Build history of the part. All positions in model axes, mm. A direction names the side the tool comes from. Round coordinates to 2 decimals unless told otherwise and drop trailing zeros. Loops run counter-clockwise (first coordinate to the right, second up) from the corner with the lowest first, then second, coordinate; pieces in that order, holes last. Notation, with made-up numbers: (45, 37.25) - (59, 37.25) arc R26 cw to (59, 59.25) - close; hole circle Ø3 at (88.5, -11.5). An arc over 180 degrees is marked (long way). Use a Markdown table: item, result.
from build123d import *

# Parameters (mm, degrees)
BOSS_EXTRUDE1_DEPTH = 10
SKETCH3_R           = 2.9999999999999973
CUT_EXTRUDE1_DEPTH  = 10
FILLET3_R           = 2
SKETCH4_R           = 1.4999999999999998
CUT_EXTRUDE2_DEPTH  = 10
SKETCH5_R           = 1.5000000000000002
CUT_EXTRUDE3_DEPTH  = 10


with BuildPart() as part:
    # Sketch2 → Boss-Extrude1 (new body)
    with BuildSketch(Plane(origin=(0, 0, 0), x_dir=(1, 0, 0), z_dir=(0, 1, 0))):
        Polygon((32.000000000000014, -27.000000000000004), (39.000000000000014, -27.000000000000004), (39.00000000000001, 18.000000000000004), (-18, 18), (-18, -13), (-12.999999999999998, -13), (-12.999999999999998, 13), (13.000000000000002, 13), (32, 13), align=None)
    extrude(amount=BOSS_EXTRUDE1_DEPTH)

    # Sketch3 → Cut-Extrude1 (cut)
    with BuildSketch(Plane(origin=(39.00000000000001, 0, -6.01e-15), x_dir=(0, 0, -1), z_dir=(1, 0, 0))):
        with Locations((-21, 5)):
            Circle(SKETCH3_R)
    extrude(amount=-CUT_EXTRUDE1_DEPTH, mode=Mode.SUBTRACT)

    # Fillet3
    fillet3_edges = [part.edges().sort_by_distance(p)[0] for p in [
        (-15.5, 0, 13),
        (-18, 0, -2.5),
        (10.500000000000004, 0, -18),
        (39.000000000000014, 0, 4.5),
        (35.500000000000014, 0, 27.000000000000004),
        (10.500000000000004, 10, -18),
        (-18, 5, 13),
        (-18, 5, -18),
        (39.00000000000001, 5, -18.000000000000004),
        (39.000000000000014, 5, 27.000000000000004),
        (-18, 10, -2.5),
        (-15.5, 10, 13),
        (35.500000000000014, 10, 27.000000000000004),
        (39.000000000000014, 10, 4.5),
    ]]
    fillet(fillet3_edges, radius=FILLET3_R)

    # Sketch4 → Cut-Extrude2 (cut)
    with BuildSketch(Plane(origin=(-1.1e-15, 0, -18), x_dir=(-1, 0, 6e-17), z_dir=(-6e-17, 0, -1))):
        with Locations((0.5000000000000004, 5)):
            Circle(SKETCH4_R)
    extrude(amount=-CUT_EXTRUDE2_DEPTH, mode=Mode.SUBTRACT)

    # Sketch5 → Cut-Extrude3 (cut)
    with BuildSketch(Plane.ZY.offset(18)):
        with Locations((3.47e-15, 5)):
            Circle(SKETCH5_R)
    extrude(amount=-CUT_EXTRUDE3_DEPTH, mode=Mode.SUBTRACT)


solid = part.part
Q1. Cut at C-C, the plane y = 5. List the corners of the cut face in (x, z), plus the area to 3 significant figures.
Results found:
| item | result |
|---|---|
| outline | (-18, -16) arc R2 ccw to (-16, -18) - (-2, -18) - (-2, -13) - (-13, -13) - (-13, -1.5) - (-18, -1.5) - close; (-18, 1.5) - (-13, 1.5) - (-13, 13) - (-16, 13) arc R2 ccw to (-18, 11) - close; (1, -18) - (37, -18) arc R2 ccw to (39, -16) - (39, 18) - (32, 18) - (32, -13) - (1, -13) - close; (32, 24) - (39, 24) - (39, 25) arc R2 ccw to (37, 27) - (32, 27) - close |
| area | 620 mm2 |
Q2. Cut at A-A, the plane z = -3.5. List the corners of the cut face in (x, y).
Results found:
| item | result |
|---|---|
| outline | (-18, 2) arc R2 ccw to (-16, 0) - (-13, 0) - (-13, 10) - (-16, 10) arc R2 ccw to (-18, 8) - close; (32, 0) - (37, 0) arc R2 ccw to (39, 2) - (39, 8) arc R2 ccw to (37, 10) - (32, 10) - close |
Q3. Probe line 1 (X direction, y = 6, z = 6); line 2 (Z direction, x = 16.5, y = 4.75); line 3 (X direction, y = 2.5, z = 19). List the from-to ranges inside material, lowest first.
Results found:
| item | result |
|---|---|
| line 1 | x = -18 to -13, 32 to 39 |
| line 2 | z = -18 to -13 |
| line 3 | x = 32 to 39 |
Q4. Drop flat-ended pins along their axis: pin 1 (6 mm diameter, centred on x = -7, z = -8.5, fed in from +Y); pin 2 (2.5 mm diameter, centred on x = -14.5, y = 5.5, fed in from +Z); pin 3 (2 mm diameter, centred on y = 3.5, z = 13, fed in from -X); pin 4 (5 mm diameter, centred on x = 15, y = 3.5, fed in from +Z). Give the stop position or say it passes through.
Results found:
| item | result |
|---|---|
| pin 1 | passes through |
| pin 2 | stops at z = 13 |
| pin 3 | stops at x = -17.73 |
| pin 4 | stops at z = -13 |
Q5. Which spindle directions (+Z, -Z, +X, -X, +Y, -Y) get a long thin tool onto all of the face, cutting with end or side? Do faces 1 (the face through (-15.5, 4.1, -1.2)), 2 (the face through (36, 5, 24)), 3 (the face through (38.43, 0.6, 4.21)), 4 (the face through (9, 5, -13)), 5 (the face through (-15, 5, 13)). Say none if no direction does.
Results found:
| item | result |
|---|---|
| face 1 | -X |
| face 2 | +X, -X |
| face 3 | +Z, -Z, +X, -Y |
| face 4 | +Z, +Y, -Y |
| face 5 | +Z, -X, +Y, -Y |
Q6. Cut at B-B, the plane x = 33. List the corners of the cut face in (y, z), plus the area to 3 significant figures.
Results found:
| item | result |
|---|---|
| outline | (0, -16) arc R2 ccw to (2, -18) - (8, -18) arc R2 ccw to (10, -16) - (10, 25) arc R2 ccw to (8, 27) - (2, 27) arc R2 ccw to (0, 25) - close; hole circle Ø6 at (5, 21) |
| area | 418 mm2 |
Q7. Pull direction X, two halves, no side cores. Call faces 6 (the face through (38.43, 9.4, 4.21)), 7 (the face through (-17.43, 5.04, 12.4)), 8 (the face through (-13, 3, 0)), 9 (the face through (14, 10, -14)): pulls with the +X half, pulls with the -X half, needs draft (parallel to the pull), parting line crosses it, or undercut.
Results found:
| item | result |
|---|---|
| face 6 | pulls with the +X half |
| face 7 | pulls with the -X half |
| face 8 | undercut |
| face 9 | needs draft |
Q8. Cut at D-D, the plane x = -0.5. List the corners of the cut face in (y, z).
Results found:
| item | result |
|---|---|
| outline | (0, -16) arc R2 ccw to (2, -18) - (3.5, -18) - (3.5, -13) - (0, -13) - close; (6.5, -18) - (8, -18) arc R2 ccw to (10, -16) - (10, -13) - (6.5, -13) - close |
